For this review, take the finished solid that the model builds, in its own axes (mm). Face numbers are marked on the shaded views. A direction names the side the tool comes from. Coordinates: 2 decimals unless noted, no trailing zeros. Write each loop counter-clockwise with the first axis right and the second up, starting at its lowest first coordinate (ties: lowest second). Pieces come first, ordered by that corner, then holes. Notation, with made-up numbers: M 2,50.5 L 14,50.5 A34 cw 14,80.5 Z; hole C -19,55.5 d10. An arc over 180 degrees is marked long. One line per question, with ' | ' between items.
from build123d import *

# Parameters (mm, degrees)
SKETCH1_R           = 69.55
BOSS_EXTRUDE1_DEPTH = 3
SKETCH2_R           = 72.55
SKETCH2_R_2         = 66.55
BOSS_EXTRUDE2_DEPTH = 3
SKETCH4_R           = 3.5
SKETCH4_R_2         = 1.45
BOSS_EXTRUDE3_DEPTH = 13
SKETCH5_R           = 3.15
BOSS_EXTRUDE4_DEPTH = 3
CIRPATTERN1_COUNT   = 4
SKETCH6_R           = 27.5
BOSS_EXTRUDE5_DEPTH = 20
SKETCH7_R           = 12
CUT_EXTRUDE1_DEPTH  = 128.58450141
SKETCH8_R           = 24
CUT_EXTRUDE2_DEPTH  = 18
SKETCH9_R           = 2.4
CUT_EXTRUDE3_DEPTH  = 127.264820912
SKETCH10_W          = 19.93582071
SKETCH10_H          = 6.3
SKETCH10_W_2        = 6.3
SKETCH10_H_2        = 19.93582071
CUT_EXTRUDE4_DEPTH  = 126.131151197


with BuildPart() as part:
    # Sketch1 → Boss-Extrude1 (new body)
    with BuildSketch(Plane(origin=(0, 0, 0), x_dir=(1, 0, 0), z_dir=(0, 1, 0))):
        with Locations(Location((0, 0, 0), (0, 0, 270))):
            Circle(SKETCH1_R)
    extrude(amount=BOSS_EXTRUDE1_DEPTH)

    # Sketch2 → Boss-Extrude2 (add)
    with BuildSketch(Plane(origin=(0, 3, 0), x_dir=(1, 0, 0), z_dir=(0, 1, 0))):
        with Locations(Location((0, 0, 0), (0, 0, 270))):
            Circle(SKETCH2_R)
        with Locations(Location((0, 0, 0), (0, 0, 270))):
            Circle(SKETCH2_R_2, mode=Mode.SUBTRACT)
    extrude(amount=BOSS_EXTRUDE2_DEPTH)

    # Sketch4 → Boss-Extrude3 (add)
    # profile 1 of 4: a face of its own
    with BuildSketch(Plane(origin=(0, 3, 0), x_dir=(1, 0, 0), z_dir=(0, 1, 0))):
        with Locations(Location((-28.75, 46, 0), (0, 0, 270))):
            Circle(SKETCH4_R)
        with Locations(Location((-28.75, 46, 0), (0, 0, 270))):
            Circle(SKETCH4_R_2, mode=Mode.SUBTRACT)
    # profile 2 of 4: a face of its own
    with BuildSketch(Plane(origin=(0, 3, 0), x_dir=(1, 0, 0), z_dir=(0, 1, 0))):
        with Locations(Location((33.75, 19.25, 0), (0, 0, 270))):
            Circle(SKETCH4_R)
        with Locations(Location((33.75, 19.25, 0), (0, 0, 270))):
            Circle(SKETCH4_R_2, mode=Mode.SUBTRACT)
    # profile 3 of 4: a face of its own
    with BuildSketch(Plane(origin=(0, 3, 0), x_dir=(1, 0, 0), z_dir=(0, 1, 0))):
        with Locations(Location((30.25, -45.75, 0), (0, 0, 270))):
            Circle(SKETCH4_R)
        with Locations(Location((30.25, -45.75, 0), (0, 0, 270))):
            Circle(SKETCH4_R_2, mode=Mode.SUBTRACT)
    # profile 4 of 4: a face of its own
    with BuildSketch(Plane(origin=(0, 3, 0), x_dir=(1, 0, 0), z_dir=(0, 1, 0))):
        with Locations(Location((-45.5, -45.25, 0), (0, 0, 176.546315789))):
            Circle(SKETCH4_R)
        with Locations(Location((-45.5, -45.25, 0), (0, 0, 270))):
            Circle(SKETCH4_R_2, mode=Mode.SUBTRACT)
    extrude(amount=BOSS_EXTRUDE3_DEPTH)

    # Sketch5 → Boss-Extrude4 (add)
    with BuildSketch(Plane(origin=(0, 3, 0), x_dir=(1, 0, 0), z_dir=(0, 1, 0))):
        with BuildLine():
            Line((-9, -69.55), (9, -69.55))
            Line((9, -69.55), (9, -77.55))
            ThreePointArc((9, -77.55), (0, -86.55), (-9, -77.55))
            Line((-9, -77.55), (-9, -69.55))
        make_face()
        with Locations(Location((0, -79, 0), (0, 0, 270))):
            Circle(SKETCH5_R, mode=Mode.SUBTRACT)
    boss_extrude4 = extrude(amount=BOSS_EXTRUDE4_DEPTH)

    # CirPattern1: Boss-Extrude4 ×4 about axis
    cirpattern1_axis = Axis((0, 0, 0), (0, 1, 0))
    for i in range(1, CIRPATTERN1_COUNT):
        add(boss_extrude4.rotate(cirpattern1_axis, i * 360 / CIRPATTERN1_COUNT))

    # Sketch6 → Boss-Extrude5 (add)
    with BuildSketch(Plane.XZ):
        with Locations(Location((0, 0, 0), (0, 0, 270))):
            Circle(SKETCH6_R)
    extrude(amount=BOSS_EXTRUDE5_DEPTH)

    # Sketch7 → Cut-Extrude1 (cut, through all)
    with BuildSketch(Plane.XZ.offset(20)):
        with Locations(Location((0, 0, 0), (0, 0, 270))):
            Circle(SKETCH7_R)
    extrude(amount=-CUT_EXTRUDE1_DEPTH, mode=Mode.SUBTRACT)

    # Sketch8 → Cut-Extrude2 (cut)
    with BuildSketch(Plane(origin=(0, 3, 0), x_dir=(1, 0, 0), z_dir=(0, 1, 0))):
        with Locations(Location((0, 0, 0), (0, 0, 270))):
            Circle(SKETCH8_R)
    extrude(amount=-CUT_EXTRUDE2_DEPTH, mode=Mode.SUBTRACT)

    # Sketch9 → Cut-Extrude3 (cut, through all)
    with BuildSketch(Plane(origin=(0, -15, 0), x_dir=(1, 0, 0), z_dir=(0, 1, 0))):
        with Locations(Location((0, 17.41, 0), (0, 0, 270))):
            Circle(SKETCH9_R)
        with Locations(Location((-15.07750228, -8.705, 0), (0, 0, 270))):
            Circle(SKETCH9_R)
        with Locations(Location((15.07750228, -8.705, 0), (0, 0, 270))):
            Circle(SKETCH9_R)
    extrude(amount=-CUT_EXTRUDE3_DEPTH, mode=Mode.SUBTRACT)

    # Sketch10 → Cut-Extrude4 (cut, through all)
    with BuildSketch(Plane(origin=(0, 6, 0), x_dir=(1, 0, 0), z_dir=(0, 1, 0))):
        with Locations((-88.967910355, 0)):
            Rectangle(SKETCH10_W, SKETCH10_H)
        with Locations((0, -88.967910355)):
            Rectangle(SKETCH10_W_2, SKETCH10_H_2)
        with Locations((88.967910355, 0)):
            Rectangle(SKETCH10_W, SKETCH10_H)
    extrude(amount=-CUT_EXTRUDE4_DEPTH, mode=Mode.SUBTRACT)

    # Sketch11 → Revolve1 (revolve)
    with BuildSketch(Plane(origin=(0, 0, 0), x_dir=(0, 0, -1), z_dir=(1, 0, 0))):
        with BuildLine():
            Line((27.5, 0), (27.5, -5))
            ThreePointArc((27.5, -5), (31.035533906, -3.535533906), (32.5, 0))
            Line((32.5, 0), (27.5, 0))
        make_face()
    revolve(axis=Axis((0, -20, 0), (0, 1, 0)))


solid = part.part
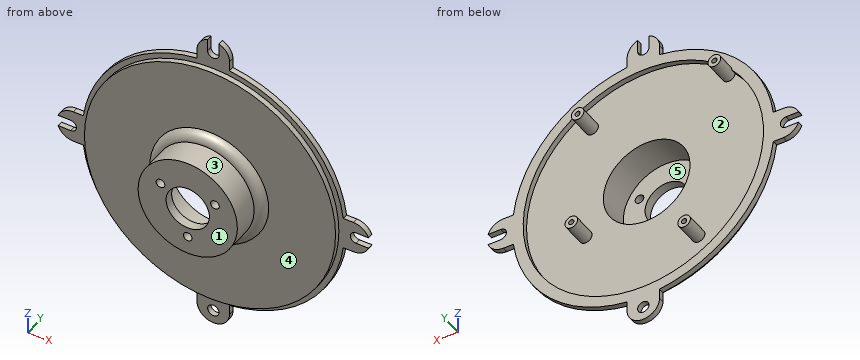
1. For line 1 along Z through (x, y) = (30, 8); line 2 along Y through (x, z) = (-34.5, 34); line 3 along Z through (x, y) = (12, -3.5), list the stretches that pass through material, from the lowest coordinate up.
Computed values:
line 1: z = 42.26 to 44.32, 47.18 to 49.24 | line 2: y = 0 to 3 | line 3: z = -28.66 to -20.78, 20.78 to 28.66
2. Draft analysis for pull direction Z (two halves, no side actions). For the marked faces 1, 2 and 3, state which applies: pulls with the +Z half, pulls with the -Z half, needs draft (parallel to the pull), parting line crosses it, or undercut.
Computed values:
face 1: needs draft | face 2: undercut | face 3: parting line crosses it
3. Take a section at A-A on x = -58.5. State the section outline as (y, z) points, plus the area to 3 significant figures.
Computed values:
outline: M 0,-37.62 L 3,-37.62 L 3,-42.91 L 6,-42.91 L 6,-31.73 L 3,-31.73 L 3,31.73 L 6,31.73 L 6,42.91 L 3,42.91 L 3,37.62 L 0,37.62 Z | area: 293 mm2
4. Take a section at B-B on y = -9. State the section outline as (x, z) points.
Computed values:
outline: C 0,0 d55; hole C 0,0 d48
5. Take a section at C-C on x = 44. State the section outline as (y, z) points.
Computed values:
outline: M 0,-53.86 L 3,-53.86 L 3,-57.68 L 6,-57.68 L 6,-49.93 L 3,-49.93 L 3,49.93 L 6,49.93 L 6,57.68 L 3,57.68 L 3,53.86 L 0,53.86 Z
6. Clearance check with flat-ended pins moving along their axes: P1, Ø0.9, axis at y = 4.5, z = -74, coming from the +X side; P2, Ø3.5, axis at y = 4.5, z = 74, coming from the -X side; P3, Ø6, axis at x = -15.08, z = 8.7, coming from the +Y side; P4, Ø6, axis at y = 11.5, z = -68.5, coming from the +X side. State where each tip first meets the part, or that it passes through.
Computed values:
P1: stops at x = 9 | P2: stops at x = -9 | P3: stops at y = -15 | P4: passes through
7. Machinability: for the marked faces 4 and 5, which of the approach directions +Z, -Z, +X, -X, +Y, -Y give a long, thin tool a straight path to every point of the face, cutting with its end or side? Answer none if there is none.
Computed values:
face 4: -Y | face 5: +Y
